Could you check a few things on this model? Use its own coordinates, in mm. A direction names the side the tool comes from. Round coordinates to 2 decimals unless told otherwise and drop trailing zeros. Loops run counter-clockwise (first coordinate to the right, second up) from the corner with the lowest first, then second, coordinate; pieces in that order, holes last. Notation, with made-up numbers: (68.5, 37.25) - (118.5, 37.25) arc R35 cw to (118.5, 71.25) - close; hole circle Ø3 at (5, -19.5). An arc over 180 degrees is marked (long way). Put each result on its own line as item: value. Start each with the question number.
from build123d import *

# Parameters (mm, degrees)
F0_W     = 260.748
F0_H     = 147.25
F0_R     = 4
F0_R_2   = 7.5
F0_W_2   = 84.36
F0_H_2   = 30
F0_W_3   = 109.668
F0_H_3   = 7.5
F1_DEPTH = 15


with BuildPart() as f1:
    # F0 (on Top) → F1 (new body)
    with BuildSketch(Plane.XY):
        with Locations((130.374, 73.625)):
            Rectangle(F0_W, F0_H)
        with Locations((12, 12)):
            Circle(F0_R, mode=Mode.SUBTRACT)
        with Locations((57.5, 65)):
            Circle(F0_R_2, mode=Mode.SUBTRACT)
        with Locations((248.748, 12)):
            Circle(F0_R, mode=Mode.SUBTRACT)
        with Locations((143.26, 65)):
            Rectangle(F0_W_2, F0_H_2, mode=Mode.SUBTRACT)
        with Locations((12, 135.25)):
            Circle(F0_R, mode=Mode.SUBTRACT)
        with Locations((155.914, 93.5)):
            Rectangle(F0_W_3, F0_H_3, mode=Mode.SUBTRACT)
        with Locations((248.748, 135.25)):
            Circle(F0_R, mode=Mode.SUBTRACT)
    extrude(amount=F1_DEPTH)


solid = f1.part
Item 1: I need wall thicknesses on line 1 (Y direction, x = 161, z = 13.25); line 2 (Y direction, x = 12, z = 11.25); line 3 (Y direction, x = 199.5, z = 8.5). Which ranges of each line are inside material? Lowest first, please. Write a range as from..to.
Item 2: Suppose I cut it at C-C, the plane x = 57.5. List the corners of the cut face in (y, z) for me.
Item 3: Thinking about a two-plate mould opening in Y: for faces 1 (the face through (100, 75, 15)), 2 (the face through (129, 147.25, 7)), 3 (the face through (52, 70.1, 7.4)), which applies, released by +Y, released by -Y, zero draft, split by the parting line, or undercut?
Item 4: Suppose I cut it at B-B, the plane z = 3.5. List the corners of the cut face in (x, y) for me, then the cut area to 3 significant figures.
Item 5: Suppose I cut it at A-A, the plane y = 135.25. List the corners of the cut face in (x, z) for me, then the cut area to 3 significant figures.
Item 6: On a 3-axis mill with a long thin cutter (end or side, diameter ignored), from which of +Z, -Z, +X, -X, +Y, -Y can I reach the whole of each face in a straight line? I mean faces 4 (the face through (155, 97.25, 7)), 5 (the face through (0, 73, 7)). Say none if no direction works.
Item 7: Suppose I cut it at D-D, the plane y = 75.5. List the corners of the cut face in (x, z) for me, then the cut area to 3 significant figures.
Item 8: Will these pins go through, and if not, where does the flat tip stop? P1, Ø1, axis at x = 152, z = 13, coming from the -Y side; P2, Ø6.5, axis at x = 12, y = 12, coming from the +Z side.
Numbers:
1. line 1: 0..50, 80..89.75, 97.25..147.25
1. line 2: 0..8, 16..131.25, 139.25..147.25
1. line 3: 0..89.75, 97.25..147.25
2. outline: (0, 0) - (57.5, 0) - (57.5, 15) - (0, 15) - close; (72.5, 0) - (147.25, 0) - (147.25, 15) - (72.5, 15) - close
3. face 1: zero draft
3. face 2: released by +Y
3. face 3: undercut
4. outline: (0, 0) - (260.75, 0) - (260.75, 147.25) - (0, 147.25) - close; hole circle Ø8 at (12, 12); hole circle Ø8 at (12, 135.25); hole circle Ø15 at (57.5, 65); hole (101.08, 50) - (185.44, 50) - (185.44, 80) - (101.08, 80) - close; hole (101.08, 89.75) - (210.75, 89.75) - (210.75, 97.25) - (101.08, 97.25) - close; hole circle Ø8 at (248.75, 12); hole circle Ø8 at (248.75, 135.25)
4. area: 34,700 mm^2
5. outline: (0, 0) - (8, 0) - (8, 15) - (0, 15) - close; (16, 0) - (244.75, 0) - (244.75, 15) - (16, 15) - close; (252.75, 0) - (260.75, 0) - (260.75, 15) - (252.75, 15) - close
5. area: 3,670 mm^2
6. face 4: +Z, -Z
6. face 5: +Z, -Z, -X, +Y, -Y
7. outline: (0, 0) - (101.08, 0) - (101.08, 15) - (0, 15) - close; (185.44, 0) - (260.75, 0) - (260.75, 15) - (185.44, 15) - close
7. area: 2,650 mm^2
8. P1: y = 0
8. P2: through
